from build123d import *

# Parameters (mm, degrees)
SKETCH1_R           = 4
BOSS_EXTRUDE1_DEPTH = 2.5
SKETCH2_R           = 4
BOSS_EXTRUDE2_DEPTH = 2.5
SKETCH3_W           = 5
SKETCH3_H           = 15
CUT_EXTRUDE1_DEPTH  = 5


with BuildPart() as part:
    # Sketch1 → Boss-Extrude1 (new, symmetric)
    with BuildSketch(Plane.XY):
        Polygon((28, 137), (-28, 137), (-28, 90), (-23, 90), (-23, 70), (-28, 70), (-28, -70), (-23, -70), (-23, -90), (-28, -90), (-28, -137), (28, -137), (28, -90), (23, -90), (23, -70), (28, -70), (28, 70), (23, 70), (23, 90), (28, 90), align=None)
        with Locations((0, -23)):
            Circle(SKETCH1_R, mode=Mode.SUBTRACT)
        with Locations((0, 57)):
            Circle(SKETCH1_R, mode=Mode.SUBTRACT)
        with Locations((0, 97)):
            Circle(SKETCH1_R, mode=Mode.SUBTRACT)
    extrude(amount=BOSS_EXTRUDE1_DEPTH, both=True)

    # Sketch2 → Boss-Extrude2 (add, symmetric)
    with BuildSketch(Plane.XY):
        with BuildLine():
            Line((144, -59), (144, -83))
            ThreePointArc((144, -83), (160, -99), (176, -83))
            Line((176, -83), (176, 23))
            Line((176, 23), (120, 23))
            Line((120, 23), (28, 23))
            Line((28, 23), (28, -9))
            Line((28, -9), (94, -9))
            ThreePointArc((94, -9), (129.355339059, -23.644660941), (144, -59))
        make_face()
        with Locations((120, 7)):
            Circle(SKETCH2_R, mode=Mode.SUBTRACT)
        with Locations((160, -43)):
            Circle(SKETCH2_R, mode=Mode.SUBTRACT)
        with Locations((160, -83)):
            Circle(SKETCH2_R, mode=Mode.SUBTRACT)
    extrude(amount=BOSS_EXTRUDE2_DEPTH, both=True)

    # Sketch3 → Cut-Extrude1 (cut)
    with BuildSketch(Plane.XY.offset(2.5)):
        with BuildLine():
            ThreePointArc((168, -83), (165.656854249, -88.656854249), (160, -91))
            Line((160, -91), (146.143593539, -91))
            ThreePointArc((146.143593539, -91), (164.141104722, -98.454813221), (176, -83))
            Line((176, -83), (176, 23))
            Line((176, 23), (144.94116403, 23))
            Line((144.94116403, 23), (144.94116403, -10.94116403))
            Line((144.94116403, -10.94116403), (168, -34))
            Line((168, -34), (168, -83))
        make_face()
        with Locations((137.5, 7)):
            Rectangle(SKETCH3_W, SKETCH3_H)
        with Locations((80, 7)):
            Rectangle(SKETCH3_W, SKETCH3_H)
    extrude(amount=-CUT_EXTRUDE1_DEPTH, mode=Mode.SUBTRACT)

    # Mirror2: part across plane


with BuildPart() as part_1:
    add(part.part)
    add(part.part.mirror(Plane(origin=(0, 0, 0), x_dir=(0, 0, 1), z_dir=(1, 0, 0))))


solid = part_1.part
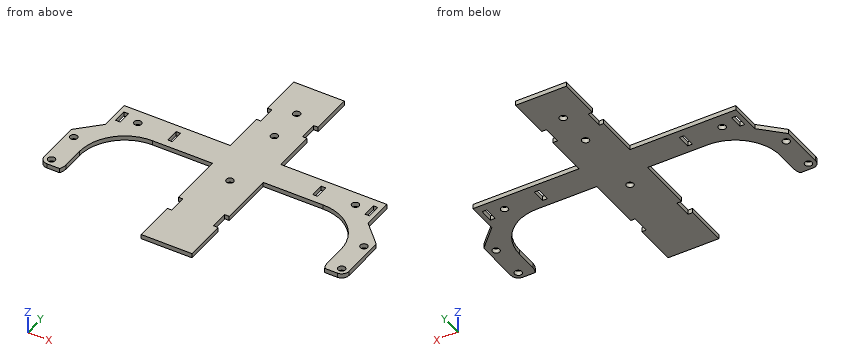
The listing builds one solid part. Answer for the finished solid, in the listing's coordinates (mm). Give positions to 0.01 mm unless a question says otherwise; leave off trailing zeros. Order: outer loops, then holes, each group sorted by start corner. A loop starts at its lowest first (then second) coordinate and runs counter-clockwise, first axis right, second up. Notation, with made-up numbers: (49, 77) - (68, 77) arc R27 ccw to (68, 110) - close; hole circle Ø1 at (45, -32.75). An arc over 180 degrees is marked (long way). Answer as CSV lines item,"result".
Q1. A cutting plane is placed at B-B, the plane y = 7. Determine the outline of the cut face in (x, z).
Answer key:
outline,"(-144.94, -2.5) - (-140, -2.5) - (-140, 2.5) - (-144.94, 2.5) - close; (-135, -2.5) - (-124, -2.5) - (-124, 2.5) - (-135, 2.5) - close; (-116, -2.5) - (-82.5, -2.5) - (-82.5, 2.5) - (-116, 2.5) - close; (-77.5, -2.5) - (77.5, -2.5) - (77.5, 2.5) - (-77.5, 2.5) - close; (82.5, -2.5) - (116, -2.5) - (116, 2.5) - (82.5, 2.5) - close; (124, -2.5) - (135, -2.5) - (135, 2.5) - (124, 2.5) - close; (140, -2.5) - (144.94, -2.5) - (144.94, 2.5) - (140, 2.5) - close"
Q2. A cutting plane is placed at C-C, the plane x = 120. Determine the outline of the cut face in (y, z), and give its area (3 significant figures).
Answer key:
outline,"(-16.29, -2.5) - (3, -2.5) - (3, 2.5) - (-16.29, 2.5) - close; (11, -2.5) - (23, -2.5) - (23, 2.5) - (11, 2.5) - close"
area,"156 mm^2"
Q3. A cutting plane is placed at D-D, the plane z = 0.8. Count the separate pieces of the cut face and the enclosed holes in it, and give its area (3 significant figures).
Answer key:
separate pieces,"1"
enclosed holes,"13"
area,"26,000 mm^2"
Q4. Each of these flat-tipped pins is pushed along its axis until it touches: pin 1 Ø1.5 at (y, z) = (96.5, -1) entering from +X; pin 2 Ø1 at (y, z) = (-1.5, 2) entering from -X; pin 3 Ø2.5 at (x, z) = (-89.5, 0.5) entering from +Y; pin 4 Ø7 at (x, y) = (0, -23) entering from -Z. Where does it stop, or does it pass through?
Answer key:
pin 1,"stops at x = 28"
pin 2,"stops at x = -144.94"
pin 3,"stops at y = 23"
pin 4,"passes through"
Q5. A cutting plane is placed at A-A, the plane y = 97. Determine the outline of the cut face in (x, z).
Answer key:
outline,"(-28, -2.5) - (-4, -2.5) - (-4, 2.5) - (-28, 2.5) - close; (4, -2.5) - (28, -2.5) - (28, 2.5) - (4, 2.5) - close"
Q6. Straight lines are drawn through the part: L1, parallel to X at y = -72, z = -1.75; L2, parallel to X at y = -35, z = -0.3; L3, parallel to Y at x = -160, z = 0.4. For each, find the intervals that lie inside material, in ascending order.
Answer key:
L1,"x = -168 to -144, -23 to 23, 144 to 168"
L2,"x = -168 to -137.86, -28 to 28, 137.86 to 168"
L3,"y = -91 to -87, -79 to -47, -39 to -26"
